Geometry: see drawing. Coordinates: mm, zero at the bounding-box minimum. Coordinates: 2 decimals unless noted, no trailing zeros. Order: outer loops, then holes, each group sorted by start corner. A loop starts at its lowest first (then second) coordinate and runs counter-clockwise, first axis right, second up. Notation, with made-up numbers: M 23.25,62.25 L 76.25,62.25 A34 cw 76.25,101.25 Z; hole C 55.5,56 d9. An arc over 180 degrees is marked long. Answer in a Markdown table with one row per item.
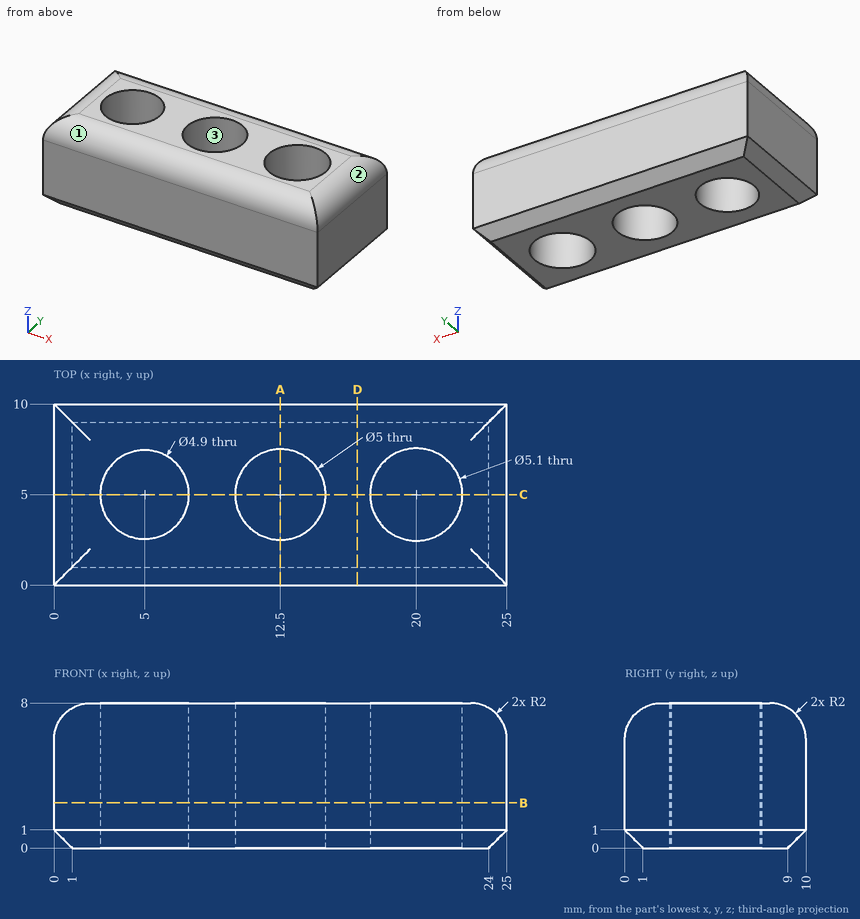
1) Cut plane A-A, the plane x = 12.5. Output: boundary loops of the cut face in (y, z), and give its area (3 significant figures).
Resolved:
| item | result |
|---|---|
| outline | M 0,1 L 1,0 L 2.5,0 L 2.5,8 L 2,8 A2 ccw 0,6 Z; M 7.5,0 L 9,0 L 10,1 L 10,6 A2 ccw 8,8 L 7.5,8 Z |
| area | 37.3 mm2 |
2) Cut plane C-C, the plane y = 5. Output: boundary loops of the cut face in (x, z).
Resolved:
| item | result |
|---|---|
| outline | M 0,1 L 1,0 L 2.55,0 L 2.55,8 L 2,8 A2 ccw 0,6 Z; M 7.45,0 L 10,0 L 10,8 L 7.45,8 Z; M 15,0 L 17.45,0 L 17.45,8 L 15,8 Z; M 22.55,0 L 24,0 L 25,1 L 25,6 A2 ccw 23,8 L 22.55,8 Z |
3) Material intervals for probe 1 along Y at (x, z) = (12.5, 5); probe 2 along X at (y, z) = (5.75, 6.5); probe 3 along X at (y, z) = (6, 0.5), sorted ascending.
Resolved:
| item | result |
|---|---|
| probe 1 | y = 0 to 2.5, 7.5 to 10 |
| probe 2 | x = 0.06 to 2.67, 7.33 to 10.12, 14.88 to 17.56, 22.44 to 24.94 |
| probe 3 | x = 0.5 to 2.76, 7.24 to 10.21, 14.79 to 17.65, 22.35 to 24.5 |
4) Cut plane D-D, the plane x = 16.75. Output: boundary loops of the cut face in (y, z).
Resolved:
| item | result |
|---|---|
| outline | M 0,1 L 1,0 L 9,0 L 10,1 L 10,6 A2 ccw 8,8 L 2,8 A2 ccw 0,6 Z |
5) Mould query, pull axis X, two halves, no side actions, for the marked faces 1, 2 and 3. Classes: +X half, -X half, draft (parallel to the pull), parting line (faces both ways), or undercut.
Resolved:
| item | result |
|---|---|
| face 1 | draft |
| face 2 | +X half |
| face 3 | undercut |
6) Contact query for a flat-ended pin moving along its axis: pin 1 (4 mm diameter, centred on x = 20, y = 5, fed in from -Z). Output: stop coordinate, or through.
Resolved:
| item | result |
|---|---|
| pin 1 | passes through |
7) Cut plane B-B, the plane z = 2.5. Output: boundary loops of the cut face in (x, y), and give its area (3 significant figures).
Resolved:
| item | result |
|---|---|
| outline | M 0,0 L 25,0 L 25,10 L 0,10 Z; hole C 5,5 d4.9; hole C 12.5,5 d5; hole C 20,5 d5.1 |
| area | 191 mm2 |
